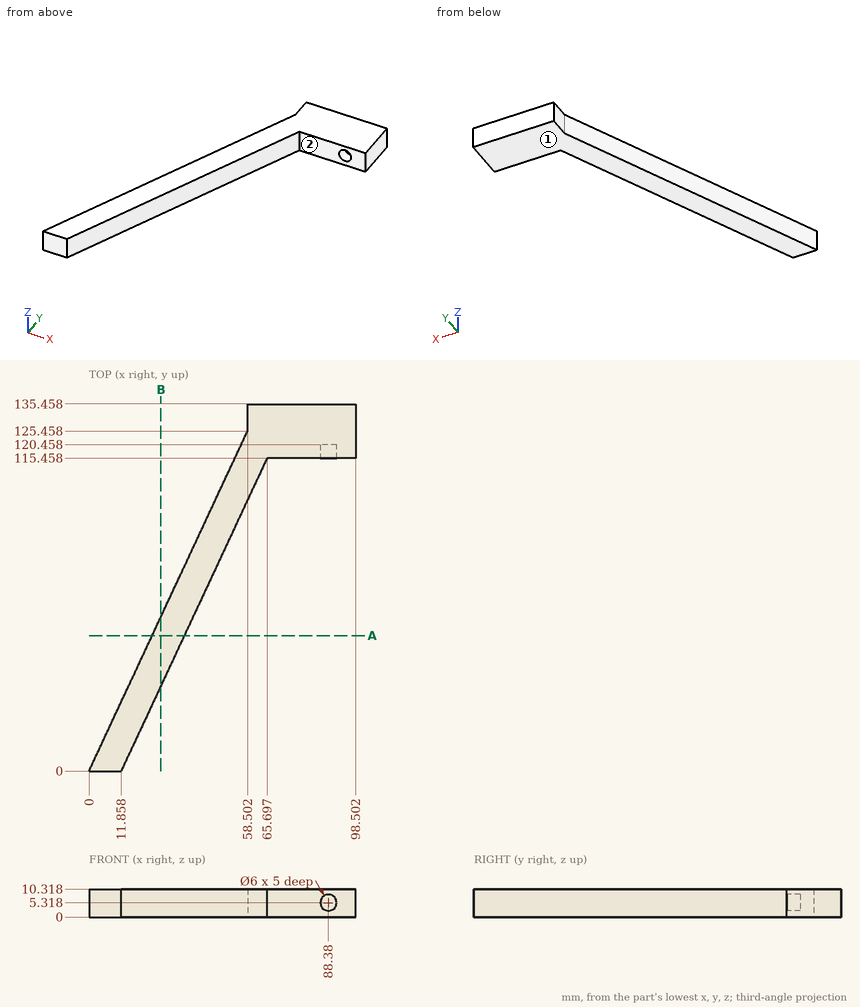
Print and shaded views of the part. All mm, measured from the part's lowest x, y and z. A direction names the side the tool comes from. Round coordinates to 2 decimals unless told otherwise and drop trailing zeros. Write each loop counter-clockwise with the first axis right and the second up, starting at its lowest first coordinate (ties: lowest second). Pieces come first, ordered by that corner, then holes. Notation, with made-up numbers: (75.5, 25) -> (79.5, 25) arc R19 cw to (79.5, 57) -> close; hole circle Ø2 at (-3, 50). An arc over 180 degrees is marked (long way). Write item = value, one per line.
(1) Band-saw the part on A-A (y = 50). Give the cut face in (x, z) (1 decimal), then the cut area to 3 significant figures.
Answer:
outline = (23.3, 0) -> (35.2, 0) -> (35.2, 10.3) -> (23.3, 10.3) -> close
area = 122 mm2
(2) Tool access for the marked faces 1 and 2: list every direction of +Z, -Z, +X, -X, +Y, -Y with a clear straight run to the whole face (end or side of a thin tool).
Answer:
face_1 = -Z, +X, -X, +Y, -Y
face_2 = +Z, -Z, +X, -Y
(3) Flat gauge pins, fed straight in: pin 1 (5 mm diameter, centred on y = 131, z = 7, fed in from -X); pin 2 (6 mm diameter, centred on x = 31.5, z = 8, fed in from -Y); pin 3 (1 mm diameter, centred on y = 55.5, z = 7, fed in from +X). Where does each tip first touch, or does it go through?
Answer:
pin_1 = 58.5
pin_2 = 35.69
pin_3 = 37.97
(4) Probe L1, parallel to Y at x = 89, z = 8.75; L2, parallel to X at y = 97, z = 5; L3, parallel to X at y = 112, z = 2.25 (1 decimal). List the from-to ranges inside material, lowest first.
Answer:
L1 = 115.46 to 135.46
L2 = 45.23 to 57.09
L3 = 52.2 to 64.1
(5) Band-saw the part on B-B (x = 26.5). Give the cut face in (y, z).
Answer:
outline = (31.4, 0) -> (56.83, 0) -> (56.83, 10.32) -> (31.4, 10.32) -> close
